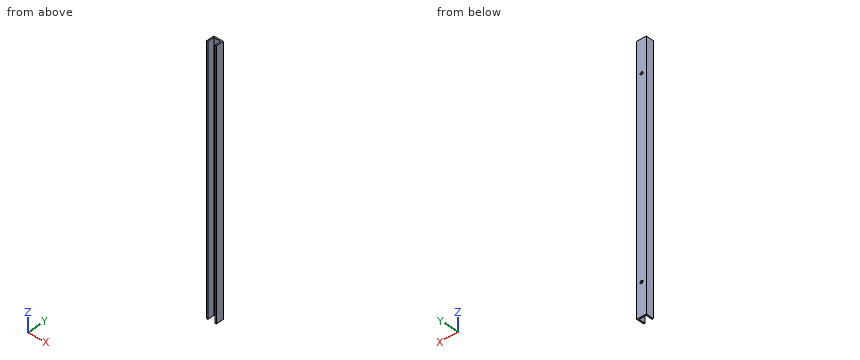
from build123d import *

# Parameters (mm, degrees)
SM_BASE_FLANGE_2_DEPTH = 402
SKETCH_7_R             = 2.25
CUT_EXTRUDE_1_DEPTH    = 403.389115161


# Sheet-metal steps are written as plain solids
with BuildPart() as part:
    # Эскиз6 → Базовая кромка2 (new body)
    with BuildSketch(Plane.XY):
        Polygon((0, 0), (-2, 0), (-2, 12), (13, 12), (13, 0), (11, 0), (11, 10), (0, 10), align=None)
    extrude(amount=-SM_BASE_FLANGE_2_DEPTH)

    # Эскиз7 → Вырез-Вытянуть1 (cut, through all)
    with BuildSketch(Plane(origin=(0, 12, 0), x_dir=(1, 0, 0), z_dir=(0, 1, 0))):
        with Locations(Location((5.5, 50, 0), (0, 0, 270))):
            Circle(SKETCH_7_R)
        with Locations(Location((5.5, 352, 0), (0, 0, 270))):
            Circle(SKETCH_7_R)
    extrude(amount=-CUT_EXTRUDE_1_DEPTH, mode=Mode.SUBTRACT)


solid = part.part
Input: part model. Units: mm. Frame: model coordinates. Give positions to 0.01 mm unless a question says otherwise; leave off trailing zeros. Loops run counter-clockwise (first coordinate to the right, second up) from the corner with the lowest first, then second, coordinate; pieces in that order, holes last. Notation, with made-up numbers: (82, 8) - (119, 8) arc R28 ccw to (119, 27) - close; hole circle Ø6 at (-32, 1). An arc over 180 degrees is marked (long way). Use CSV: the item, a comma, the result in double quotes. Start each with the question number.
Item 1: Contact query for flat-ended pins moving along their axis: P1, Ø8, axis at x = 2, z = -50.5, coming from the -Y side; P2, Ø3.5, axis at x = 5.5, z = -352, coming from the +Y side; P3, Ø3.5, axis at x = 4, z = -131, coming from the -Y side. Output: stop coordinate, or through.
Item 2: Section A-A on x = 5.5. Return loops of the section in (y, z).
Item 3: Line query: line 1 (X direction, y = 3.75, z = -365.5); line 2 (X direction, y = 11.55, z = -50); line 3 (Y direction, x = 5, z = -181). Output: solid intervals per line, ascending.
Item 4: Section B-B on y = 4.25. Return loops of the section in (x, z).
Item 5: Section C-C on z = -255. Return loops of the section in (x, y), then the cut area to 3 significant figures.
Ans:
1,P1,"stops at y = 0"
1,P2,"passes through"
1,P3,"stops at y = 10"
2,outline,"(10, -402) - (12, -402) - (12, -354.25) - (10, -354.25) - close; (10, -349.75) - (12, -349.75) - (12, -52.25) - (10, -52.25) - close; (10, -47.75) - (12, -47.75) - (12, 0) - (10, 0) - close"
3,line 1,"x = -2 to 0, 11 to 13"
3,line 2,"x = -2 to 3.25, 7.75 to 13"
3,line 3,"y = 10 to 12"
4,outline,"(-2, -402) - (0, -402) - (0, 0) - (-2, 0) - close; (11, -402) - (13, -402) - (13, 0) - (11, 0) - close"
5,outline,"(-2, 0) - (0, 0) - (0, 10) - (11, 10) - (11, 0) - (13, 0) - (13, 12) - (-2, 12) - close"
5,area,"70.0 mm2"
